CAD build for the part. Positions are in the model's coordinates, mm. Face numbers are marked on the shaded views. A direction names the side the tool comes from. Coordinates: 2 decimals unless noted, no trailing zeros. Order: outer loops, then holes, each group sorted by start corner. A loop starts at its lowest first (then second) coordinate and runs counter-clockwise, first axis right, second up. Notation, with made-up numbers: (5, 31) - (57, 31) arc R24 ccw to (57, 63) - close; hole circle Ø3 at (35, 15). An arc over 180 degrees is marked (long way). Write each question's results on one line, items separated by ' | '. Start each with the question number.
Q1. Wall check: probe 1 along X at (y, z) = (18.5, 2); probe 2 along Y at (x, z) = (26.5, 26.25); probe 3 along Y at (x, z) = (33, 20). Give the ranges that are in metal, low to high.
Q2. Which spindle directions (+Z, -Z, +X, -X, +Y, -Y) get a long thin tool onto all of the face, cutting with end or side? Do the marked faces 1, 2, 3, 4 and 5. Say none if no direction does.
Q3. Band-saw the part on A-A, the plane x = 44. Write the cut outline in (y, z), then the cut area to 3 significant figures.
Q4. Band-saw the part on C-C, the plane y = 9. Write the cut outline in (x, z).
Q5. Pull direction X, two halves, no side cores. Call the marked faces 6, 7, 8 and 9: released by +X, released by -X, zero draft, split by the parting line, or undercut.
Q6. Band-saw the part on D-D, the plane x = 26. Write the cut outline in (y, z).
Q7. Pin check, flat tips, straight feed: P1, Ø17.5, axis at x = 16, z = 18, coming from the +Y side; P2, Ø3, axis at y = 5.5, z = 19.5, coming from the -X side; P3, Ø1.2, axis at y = 17, z = 10, coming from the -X side; P4, Ø4, axis at x = 24.5, y = 29.5, coming from the +Z side. Stop position of each tip, or through.
Q8. Band-saw the part on B-B, the plane z = 24.75. Write the cut outline in (x, y).
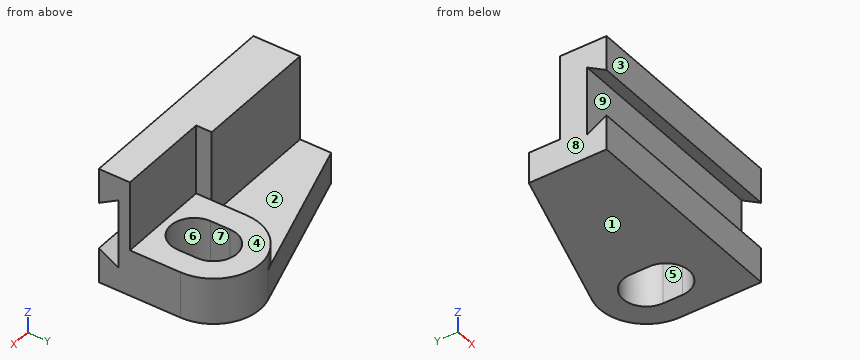
```python
from build123d import *

# Parameters (mm, degrees)
EXTRUDE_1_DEPTH     = 30
EXTRUDE_2_DEPTH     = 8
EXTRUDE_3_DEPTH     = 12
CUT_EXTRUDE_1_DEPTH = 72.589105316


with BuildPart() as part:
    # 草图1 → 凸台-拉伸1 (new body)
    with BuildSketch(Plane.XY):
        Polygon((0, 12), (0, 0), (56, 0), (56, 8), (32, 8), (32, 12), align=None)
    extrude(amount=EXTRUDE_1_DEPTH)

    # 草图1<4> → 凸台-拉伸2 (add)
    with BuildSketch(Plane.XY):
        with BuildLine():
            Line((0, 20), (0, 12))
            Line((0, 12), (32, 12))
            Line((32, 12), (32, 21))
            ThreePointArc((32, 21), (34.345975777, 28.127398986), (40.466636051, 32.468013743))
            Line((40.466636051, 32.468013743), (0, 20))
        make_face()
    extrude(amount=EXTRUDE_2_DEPTH)

    # 草图1<5> → 凸台-拉伸3 (add)
    with BuildSketch(Plane.XY):
        with BuildLine():
            Line((32, 8), (56, 8))
            Line((56, 8), (56, 21))
            ThreePointArc((56, 21), (51.127398986, 30.654024223), (40.466636051, 32.468013743))
            ThreePointArc((40.466636051, 32.468013743), (34.345975777, 28.127398986), (32, 21))
            Line((32, 21), (32, 12))
            Line((32, 12), (32, 8))
        make_face()
        with BuildLine():
            ThreePointArc((38, 21), (44, 27), (50, 21))
            Line((50, 21), (50, 16))
            ThreePointArc((50, 16), (44, 10), (38, 16))
            Line((38, 16), (38, 21))
        make_face(mode=Mode.SUBTRACT)
    extrude(amount=EXTRUDE_3_DEPTH)

    # 草图5 → 切除-拉伸1 (cut, through all)
    with BuildSketch(Plane.ZY):
        Polygon((9, 0), (6.113248654, 5), (23.886751346, 5), (21, 0), align=None)
    extrude(amount=-CUT_EXTRUDE_1_DEPTH, mode=Mode.SUBTRACT)


solid = part.part
```
Results below:
1) probe 1: x = 0 to 38, 50 to 56 | probe 2: y = 0 to 12 | probe 3: y = 5 to 8
2) face 1: -Z, +X, -X, +Y, -Y | face 2: +Z, -X, +Y | face 3: +Z, -Z, +X, -X, -Y | face 4: +Z, +X, +Y | face 5: +Z, -Z
3) outline: (0, 0) - (10, 0) - (10, 12) - (8, 12) - (8, 30) - (0, 30) - (0, 21) - (5, 23.89) - (5, 6.11) - (0, 9) - close; (27, 0) - (33, 0) - (33, 12) - (27, 12) - close | area: 262 mm²
4) outline: (0, 0) - (56, 0) - (56, 12) - (32, 12) - (32, 30) - (0, 30) - close
5) face 6: undercut | face 7: undercut | face 8: released by -X | face 9: zero draft
6) outline: (0, 0) - (28.01, 0) - (28.01, 8) - (12, 8) - (12, 30) - (0, 30) - (0, 21) - (5, 23.89) - (5, 6.11) - (0, 9) - close
7) P1: stops at y = 12 | P2: stops at x = 0 | P3: stops at x = 32 | P4: stops at z = 8
8) outline: (0, 0) - (56, 0) - (56, 8) - (32, 8) - (32, 12) - (0, 12) - close
